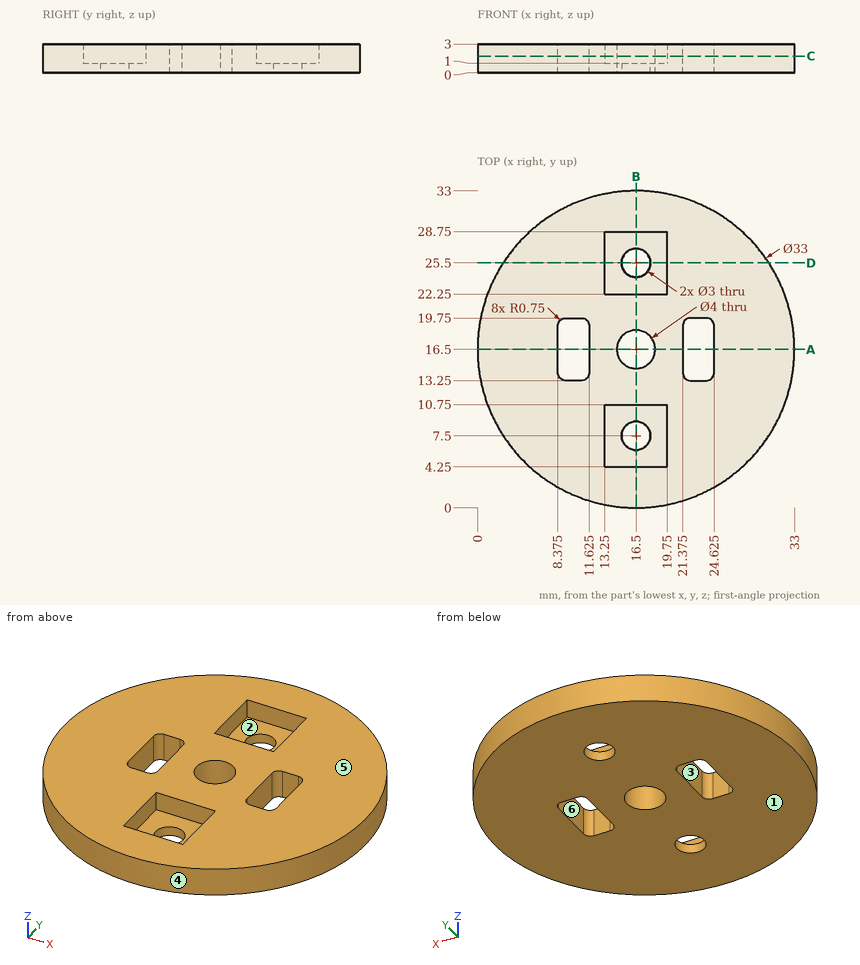
Study the drawing (mm; zero at the part's minimum x, y, z) and answer. A direction names the side the tool comes from. Give positions to 0.01 mm unless a question says otherwise; leave off trailing zeros. Loops run counter-clockwise (first coordinate to the right, second up) from the corner with the lowest first, then second, coordinate; pieces in that order, holes last. Notation, with made-up numbers: M 0.5,26.5 L 59.5,26.5 A24 cw 59.5,47.5 Z; hole C 33.5,28 d2. An arc over 180 degrees is marked long. Use CSV: the item, a comma, the result in double quotes.
1) Determine the mould class of the marked faces 4, 5 and 6 for opening direction Y: released by +Y, released by -Y, zero draft, split by the parting line, or undercut.
Answer:
face 4,"split by the parting line"
face 5,"zero draft"
face 6,"undercut"
2) Given P1, Ø0.6, axis at x = 15, z = 1.5, coming from the +Y side; P2, Ø1, axis at y = 24.5, z = 2, coming from the +X side; P3, Ø0.9, axis at x = 10, z = 1.5, coming from the +Y side; P4, Ø2.5, axis at x = 16.5, y = 7.5, coming from the +Z side, each flat-ended and moving along its own axis, determine where each tip first touches the part or whether it passes through.
Answer:
P1,"y = 32.96"
P2,"x = 31.2"
P3,"y = 31.85"
P4,"through"
3) Find section B-B on x = 16.5. Write down the section's boundary in (y, z), plus the area to 3 significant figures.
Answer:
outline,"M 0,0 L 6,0 L 6,1 L 4.25,1 L 4.25,3 L 0,3 Z; M 9,0 L 14.5,0 L 14.5,3 L 10.75,3 L 10.75,1 L 9,1 Z; M 18.5,0 L 24,0 L 24,1 L 22.25,1 L 22.25,3 L 18.5,3 Z; M 27,0 L 33,0 L 33,3 L 28.75,3 L 28.75,1 L 27,1 Z"
area,"55.0 mm^2"
4) Consider L1, parallel to Y at x = 16.5, z = 0.8; L2, parallel to Y at x = 16.5, z = 1.9; L3, parallel to X at y = 19.5, z = 0.75. Determine where each line is inside the solid, lowest interval first.
Answer:
L1,"0 to 6, 9 to 14.5, 18.5 to 24, 27 to 33"
L2,"0 to 4.25, 10.75 to 14.5, 18.5 to 22.25, 28.75 to 33"
L3,"0.28 to 8.57, 11.43 to 21.57, 24.43 to 32.72"
5) Which of the six approach directions +Z, -Z, +X, -X, +Y, -Y give full straight-line access (tool end or side, diameter ignored) to the marked faces 1, 2 and 3?
Answer:
face 1,"-Z, +X, -X, +Y, -Y"
face 2,"+Z"
face 3,"+Z, -Z"
6) Find section D-D on y = 25.5. Write down the section's boundary in (x, z).
Answer:
outline,"M 2.67,0 L 15,0 L 15,1 L 13.25,1 L 13.25,3 L 2.67,3 Z; M 18,0 L 30.33,0 L 30.33,3 L 19.75,3 L 19.75,1 L 18,1 Z"
7) Find section C-C on z = 1.75. Write down the section's boundary in (x, y) (3 decimals), plus the area to 3 significant figures.
Answer:
outline,"C 16.5,16.5 d33; hole M 8.375,14 A0.75 ccw 9.125,13.25 L 10.875,13.25 A0.75 ccw 11.625,14 L 11.625,19 A0.75 ccw 10.875,19.75 L 9.125,19.75 A0.75 ccw 8.375,19 Z; hole M 13.25,4.25 L 19.75,4.25 L 19.75,10.75 L 13.25,10.75 Z; hole M 13.25,22.25 L 19.75,22.25 L 19.75,28.75 L 13.25,28.75 Z; hole C 16.5,16.5 d4; hole M 21.375,14 A0.75 ccw 22.125,13.25 L 23.875,13.25 A0.75 ccw 24.625,14 L 24.625,19 A0.75 ccw 23.875,19.75 L 22.125,19.75 A0.75 ccw 21.375,19 Z"
area,"717 mm^2"
8) Find section A-A on y = 16.5. Write down the section's boundary in (x, z) (3 decimals), plus the area to 3 significant figures.
Answer:
outline,"M 0,0 L 8.375,0 L 8.375,3 L 0,3 Z; M 11.625,0 L 14.5,0 L 14.5,3 L 11.625,3 Z; M 18.5,0 L 21.375,0 L 21.375,3 L 18.5,3 Z; M 24.625,0 L 33,0 L 33,3 L 24.625,3 Z"
area,"67.5 mm^2"
